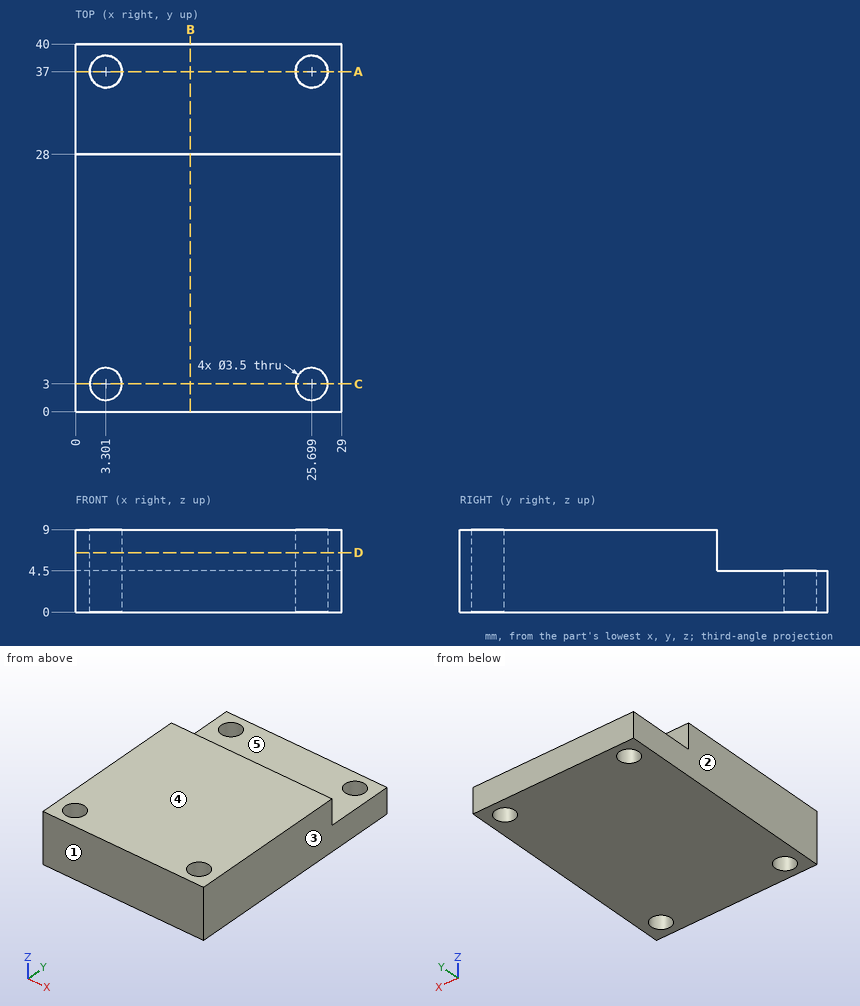
Drawing for the job (mm, zero at the part's lowest x, y, z). A direction names the side the tool comes from. Round coordinates to 2 decimals unless told otherwise and drop trailing zeros. Order: outer loops, then holes, each group sorted by start corner. A loop starts at its lowest first (then second) coordinate and runs counter-clockwise, first axis right, second up.
Item 1: Pin check, flat tips, straight feed: pin 1 (1.5 mm diameter, centred on x = 20.5, z = 3, fed in from -Y); pin 2 (3.5 mm diameter, centred on x = 12, z = 7.5, fed in from +Y); pin 3 (6 mm diameter, centred on x = 8.5, y = 33, fed in from +Z). Stop position of each tip, or through.
Item 2: Saw through at B-B on x = 12.5. Write the cut outline in (y, z).
Item 3: Saw through at A-A on y = 37. Write the cut outline in (x, z).
Item 4: Saw through at D-D on z = 6.5. Write the cut outline in (x, y).
Item 5: Tool access for the marked faces 4 and 5: list every direction of +Z, -Z, +X, -X, +Y, -Y with a clear straight run to the whole face (end or side of a thin tool).
Item 6: Probe line 1 along X through (y, z) = (37, 3.5); line 2 along Y through (x, z) = (4.5, 4.25) (1 decimal); line 3 along X through (y, z) = (4.5, 3.75) (1 decimal). List the from-to ranges inside material, lowest first.
Item 7: Saw through at C-C on y = 3. Write the cut outline in (x, z), then the cut area to 3 significant figures.
Item 8: Mould opens along X. For the marked faces 1, 2 and 3 say: pulls with the +X half, pulls with the -X half, needs draft (parallel to the pull), parting line crosses it, or undercut.
Reported:
1. pin 1: stops at y = 0
1. pin 2: stops at y = 28
1. pin 3: stops at z = 4.5
2. outline: (0, 0) - (40, 0) - (40, 4.5) - (28, 4.5) - (28, 9) - (0, 9) - close
3. outline: (0, 0) - (1.55, 0) - (1.55, 4.5) - (0, 4.5) - close; (5.05, 0) - (23.95, 0) - (23.95, 4.5) - (5.05, 4.5) - close; (27.45, 0) - (29, 0) - (29, 4.5) - (27.45, 4.5) - close
4. outline: (0, 0) - (29, 0) - (29, 28) - (0, 28) - close; hole circle Ø3.5 at (3.3, 3); hole circle Ø3.5 at (25.7, 3)
5. face 4: +Z, +X, -X, +Y, -Y
5. face 5: +Z, +X, -X, +Y
6. line 1: x = 0 to 1.55, 5.05 to 23.95, 27.45 to 29
6. line 2: y = 0 to 1.7, 4.3 to 35.7, 38.3 to 40
6. line 3: x = 0 to 2.4, 4.2 to 24.8, 26.6 to 29
7. outline: (0, 0) - (1.55, 0) - (1.55, 9) - (0, 9) - close; (5.05, 0) - (23.95, 0) - (23.95, 9) - (5.05, 9) - close; (27.45, 0) - (29, 0) - (29, 9) - (27.45, 9) - close
7. area: 198 mm2
8. face 1: needs draft
8. face 2: pulls with the -X half
8. face 3: pulls with the +X half
